Build history of the part. All positions in model axes, mm. A direction names the side the tool comes from. Round coordinates to 2 decimals unless told otherwise and drop trailing zeros. Write each loop counter-clockwise with the first axis right and the second up, starting at its lowest first coordinate (ties: lowest second). Pieces come first, ordered by that corner, then holes.
1) Wall check: probe 1 along X at (y, z) = (4, 0); probe 2 along Z at (x, y) = (11, 6.65); probe 3 along Z at (x, y) = (11, 7.2). Give the ranges that are in metal, low to high.
2) Saw through at A-A (x = 0). Write the cut outline in (y, z), plus the area to 3 significant figures.
3) Which spindle directions (+Z, -Z, +X, -X, +Y, -Y) get a long thin tool onto all of the face, cutting with end or side? Do faces 1 (the cylindrical face through (0, 3, 22)), 2 (the cylindrical face through (12.352, 6.521, -6.708)). Say none if no direction does.
4) Pull direction Z, two halves, no side cores. Call faces 3 (the cylindrical face through (0, 3, -22)), 4 (the flat face through (-20, 4, 0)), 5 (the flat face through (-11, 5, -9)): +Z half, -Z half, draft (parallel to the pull), parting line (faces both ways), or undercut.
5) Flat gauge pins, fed straight in: pin 1 (3 mm diameter, centred on x = -13.5, y = 6, fed in from -Z); pin 2 (4.5 mm diameter, centred on x = -9.5, z = -11, fed in from +Y). Where does each tip first touch, or does it go through?
6) Saw through at B-B (y = 1.25). Write the cut outline in (x, z).
7) Saw through at C-C (z = 11). State how many separate pieces and enclosed holes the cut face has, plus the area to 3 significant figures.
from build123d import *

# Parameters (mm, degrees)
SKETCH1_R                               = 22
SKETCH1_R_2                             = 8
EXTRUDE1_DEPTH                          = 8
CHAMFER1_SIZE                           = 2
CBORE_FOR_M3_HEX_HEAD_BOLT1_D           = 3.4
CBORE_FOR_M3_HEX_HEAD_BOLT1_DEPTH       = 10.1
CBORE_FOR_M3_HEX_HEAD_BOLT1_CBORE_D     = 9
CBORE_FOR_M3_HEX_HEAD_BOLT1_CBORE_DEPTH = 3
CBORE_FOR_M3_HEX_HEAD_BOLT1_TIP         = 1.021463052
SKETCH4_OUTSIDE_W                       = 58.548
SKETCH4_OUTSIDE_H                       = 58.548
SKETCH4_OUTSIDE_W_2                     = 40
SKETCH4_OUTSIDE_H_2                     = 54.265232974
EXTRUDE2_DEPTH                          = 30


with BuildPart() as part:
    # Sketch1 → Extrude1 (new body)
    with BuildSketch(Plane(origin=(0, 0, 0), x_dir=(1, 0, 0), z_dir=(0, 1, 0))):
        with Locations(Location((0, 0, 0), (0, 0, 270))):
            Circle(SKETCH1_R)
        with Locations(Location((0, 0, 0), (0, 0, 270))):
            Circle(SKETCH1_R_2, mode=Mode.SUBTRACT)
    extrude(amount=EXTRUDE1_DEPTH)

    # Chamfer1
    chamfer1_edges = [part.edges().sort_by_distance(p)[0] for p in [
        (0, 8, -22),
    ]]
    chamfer(chamfer1_edges, length=CHAMFER1_SIZE)

    # CBORE for M3 Hex Head Bolt1
    with Locations(Plane(origin=(-11, 8, -11), x_dir=(0, 0, 1), z_dir=(0, 1, 0))):
        with Locations((0, 0), (0, 22), (22, 22), (22, 0)):
            CounterBoreHole(CBORE_FOR_M3_HEX_HEAD_BOLT1_D / 2, CBORE_FOR_M3_HEX_HEAD_BOLT1_CBORE_D / 2, CBORE_FOR_M3_HEX_HEAD_BOLT1_CBORE_DEPTH, depth=CBORE_FOR_M3_HEX_HEAD_BOLT1_DEPTH)
            with Locations((0, 0, -(CBORE_FOR_M3_HEX_HEAD_BOLT1_DEPTH + CBORE_FOR_M3_HEX_HEAD_BOLT1_TIP / 2))):  # 118° drill point
                Cone(0, CBORE_FOR_M3_HEX_HEAD_BOLT1_D / 2, CBORE_FOR_M3_HEX_HEAD_BOLT1_TIP, mode=Mode.SUBTRACT)

    # Sketch4 outside → Extrude2 (cut)
    with BuildSketch(Plane.XZ):
        Rectangle(SKETCH4_OUTSIDE_W, SKETCH4_OUTSIDE_H)
        Rectangle(SKETCH4_OUTSIDE_W_2, SKETCH4_OUTSIDE_H_2, mode=Mode.SUBTRACT)
    extrude(amount=-EXTRUDE2_DEPTH, mode=Mode.SUBTRACT)


solid = part.part
Evaluation:
1. probe 1: x = -20 to -8, 8 to 20
1. probe 2: z = -18.3 to -15.5, -6.5 to 6.5, 15.5 to 18.3
1. probe 3: z = -17.65 to -15.5, -6.5 to 6.5, 15.5 to 17.65
2. outline: (0, -22) - (6, -22) - (8, -20) - (8, -8) - (0, -8) - close; (0, 8) - (8, 8) - (8, 20) - (6, 22) - (0, 22) - close
2. area: 220 mm2
3. face 1: +Z, +Y, -Y
3. face 2: +Y
4. face 3: -Z half
4. face 4: draft
4. face 5: undercut
5. pin 1: stops at z = -18.44
5. pin 2: stops at y = 5
6. outline: (-20, -9.17) arc R22 ccw to (20, -9.17) - (20, 9.17) arc R22 ccw to (-20, 9.17) - close; hole circle Ø3.4 at (-11, -11); hole circle Ø3.4 at (-11, 11); hole circle Ø16 at (0, 0); hole circle Ø3.4 at (11, -11); hole circle Ø3.4 at (11, 11)
7. separate pieces: 3
7. enclosed holes: 0
7. area: 212 mm2
